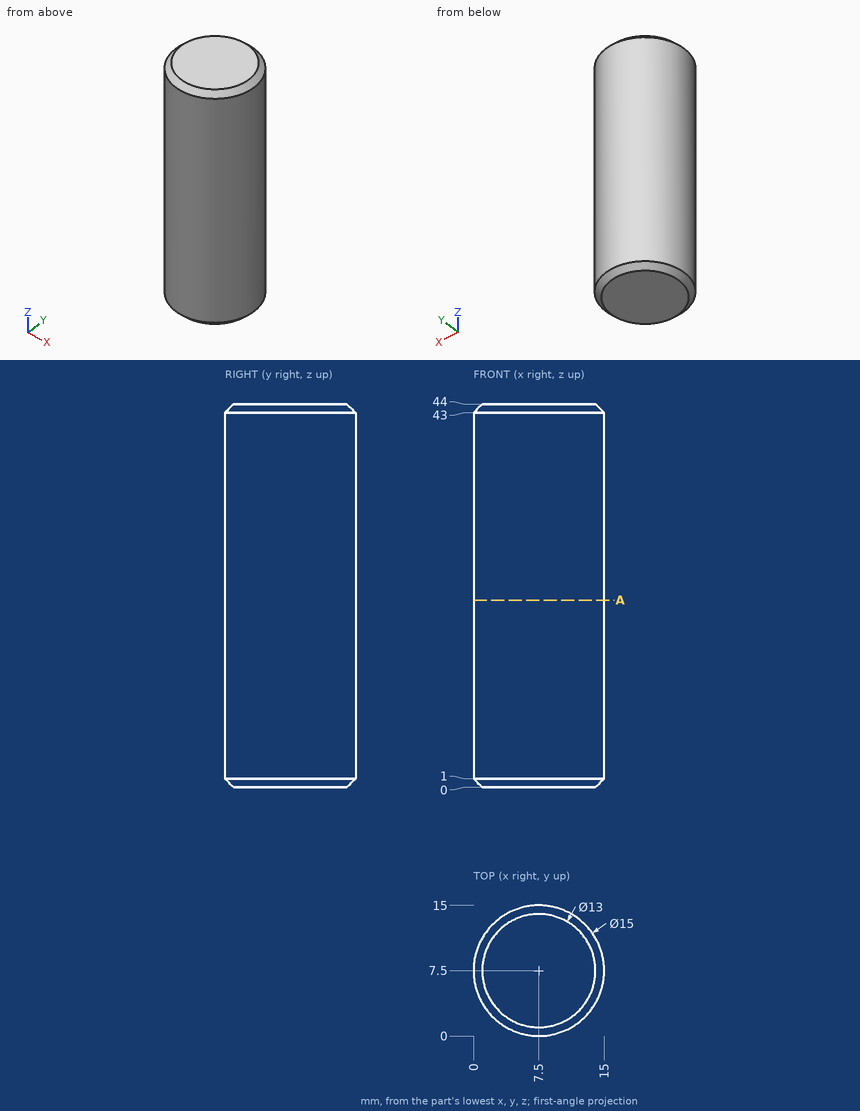
Geometry: see drawing. Coordinates: mm, zero at the bounding-box minimum. Give positions to 0.01 mm unless a question says otherwise; leave off trailing zeros. Loops run counter-clockwise (first coordinate to the right, second up) from the corner with the lowest first, then second, coordinate; pieces in that order, holes last. Notation, with made-up numbers: M -25.75,31 L -5.75,31 A18 cw -5.75,53 Z; hole C 4.25,5.5 d8. An arc over 180 degrees is marked long. Use one line per item in the form item = value.
1. First-contact query: pin 1 (1 mm diameter, centred on y = 5.5, z = 22, fed in from +X); pin 2 (6 mm diameter, centred on y = 13, z = 29.5, fed in from +X); pin 3 (5 mm diameter, centred on y = 13.5, z = 15, fed in from -X). Flat tips, straight axial feed; report the tip coordinate or a pass-through.
Numbers:
pin_1 = 14.85
pin_2 = 14.57
pin_3 = 0.87
2. Line query: L1, parallel to X at y = 3.75, z = 10; L2, parallel to X at y = 12.25, z = 7; L3, parallel to Z at x = 13.25, y = 4.25. Output: solid intervals per line, ascending.
Numbers:
L1 = 1 to 14
L2 = 1.7 to 13.3
L3 = 0.1 to 43.9
3. Section query A-A, the plane z = 21.5. Return the cut outline in (x, y), and give its area (3 significant figures).
Numbers:
outline = C 7.5,7.5 d15
area = 177 mm²
